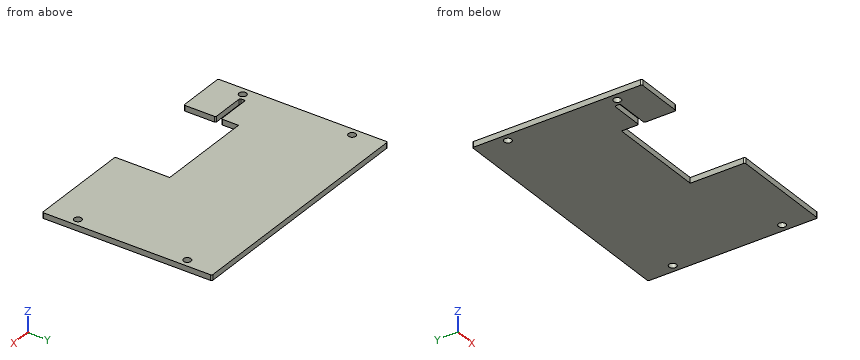
```python
from build123d import *

# Parameters (mm, degrees)
SKETCH1_W           = 145.885353282
SKETCH1_H           = 98.425
BOSS_EXTRUDE1_DEPTH = 3.2004
SKETCH4_W           = 57.100000132
SKETCH4_H           = 31.75
CUT_EXTRUDE1_DEPTH  = 3.2004
SKETCH5_R           = 2.159
CUT_EXTRUDE2_DEPTH  = 3.2004
SKETCH7_W           = 20.092850022
SKETCH7_H           = 3.175
CUT_EXTRUDE4_DEPTH  = 3.2004
FILLET1_R           = 0.762


with BuildPart() as part:
    # Sketch1 → Boss-Extrude1 (new body)
    with BuildSketch(Plane.XY):
        with Locations((72.942676641, 49.2125)):
            Rectangle(SKETCH1_W, SKETCH1_H)
    extrude(amount=BOSS_EXTRUDE1_DEPTH)

    # Sketch4 → Cut-Extrude1 (cut)
    with BuildSketch(Plane.XY.offset(3.2004)):
        with Locations((56.982760066, 15.875)):
            Rectangle(SKETCH4_W, SKETCH4_H)
    extrude(amount=-CUT_EXTRUDE1_DEPTH, mode=Mode.SUBTRACT)

    # Sketch5 → Cut-Extrude2 (cut)
    with BuildSketch(Plane.XY.offset(3.2004)):
        with Locations((141.376853282, 80.9625)):
            Circle(SKETCH5_R)
        with Locations((141.376853282, 17.4625)):
            Circle(SKETCH5_R)
        with Locations((4.5085, 17.4625)):
            Circle(SKETCH5_R)
        with Locations((4.5085, 80.9625)):
            Circle(SKETCH5_R)
    extrude(amount=-CUT_EXTRUDE2_DEPTH, mode=Mode.SUBTRACT)

    # Sketch7 → Cut-Extrude4 (cut)
    with BuildSketch(Plane(origin=(0, 0, 0), x_dir=(-1, 0, 0), z_dir=(0, 0, -1))):
        with Locations((-18.386334989, 20.09902)):
            Rectangle(SKETCH7_W, SKETCH7_H)
    extrude(amount=-CUT_EXTRUDE4_DEPTH, mode=Mode.SUBTRACT)

    # Fillet1
    fillet1_edges = [part.edges().sort_by_distance(p)[0] for p in [
        (28.43276, 0, 1.6002),
        (85.532760132, 0, 1.6002),
        (8.339909978, 18.51152, 1.6002),
        (8.339909978, 21.68652, 1.6002),
        (28.43276, 21.68652, 1.6002),
        (28.43276, 18.51152, 1.6002),
        (0, 98.425, 1.6002),
        (145.885353282, 98.425, 1.6002),
        (145.885353282, 0, 1.6002),
        (0, 0, 1.6002),
    ]]
    fillet(fillet1_edges, radius=FILLET1_R)


solid = part.part
```
Geometry: final body of the model. Coordinates: model frame, mm. Round coordinates to 2 decimals unless told otherwise and drop trailing zeros. Loops run counter-clockwise (first coordinate to the right, second up) from the corner with the lowest first, then second, coordinate; pieces in that order, holes last. Notation, with made-up numbers: (21, 15.5) -> (64, 15.5) arc R22 ccw to (64, 41.5) -> close; hole circle Ø11 at (84.5, 22.5). An arc over 180 degrees is marked (long way). Use one line per item in the form item = value. Start each with the question number.
1) First-contact query: P1, Ø2.5, axis at x = 141.38, y = 17.46, coming from the +Z side. Flat tip, straight axial feed; report the tip coordinate or a pass-through.
2) Section A-A on z = 1.4. Give the number of separate pieces and of enclosed holes in the cut face, then the cut area to 3 significant figures.
3) Line query: L1, parallel to X at y = 12.5, z = 1.25; L2, parallel to Y at x = 49, z = 1.1 (3 decimals). Output: solid intervals per line, ascending.
4) Section B-B on x = 64. Output: boundary loops of the cut face in (y, z) (3 decimals).
Response:
q1.P1 = through
q2.separate_pieces = 1
q2.enclosed_holes = 4
q2.area = 12,400 mm^2
q3.L1 = 0 to 28.43, 85.53 to 145.89
q3.L2 = 31.75 to 98.425
q4.outline = (31.75, 0) -> (98.425, 0) -> (98.425, 3.2) -> (31.75, 3.2) -> close
